Source: CAD feature listing. Evaluate the final solid. Frame: model axes, mm. A direction names the side the tool comes from. Give positions to 0.01 mm unless a question says otherwise; leave off trailing zeros. Write each loop counter-clockwise with the first axis right and the second up, starting at its lowest first coordinate (ties: lowest second). Pieces come first, ordered by that corner, then holes. Notation, with made-up numbers: (68.5, -3) -> (80.5, -3) arc R14 ccw to (80.5, 9) -> close; hole circle Ø3 at (16, 55.5). An arc over 180 degrees is marked (long way). Use one line per item in the form item = value. Start each with the question number.
(1) Cut plane B-B, the plane x = 17.5. Output: boundary loops of the cut face in (y, z), and give its area (3 significant figures).
(2) Draft query along X for faces 4 (the face through (9.56, -6.68, -6.08)), 5 (the face through (26.745, 6.2, 0.1)), 6 (the face through (69.486, -10.648, -13.887)). Return one class per face: pulls with the +X half, pulls with the -X half, needs draft (parallel to the pull), parting line crosses it, or undercut.
(3) Set-up query: faces 1 (the face through (58.381, 0.66, -14.985)), 2 (the face through (50.45, 8.43, 5.38)), 3 (the face through (3.226, 14.756, 9.408)). Return all of +Z, -Z, +X, -X, +Y, -Y with unobstructed straight access to the full face (end or side cutting, diameter ignored); none if empty.
(4) Cut plane A-A, the plane x = 55. Output: boundary loops of the cut face in (y, z).
(5) Material intervals for line 1 along Y through (x, z) = (59, 0); line 2 along X through (y, z) = (-12.5, -7); line 3 along Y through (x, z) = (47.5, 6.5), sorted ascending. Write a range as from..to.
(6) First-contact query: P1, Ø10, axis at x = 64.5, y = 5, coming from the +Z side; P2, Ø6.5, axis at x = 29.5, z = 2, coming from the +Y side; P3, Ø18, axis at x = 17.5, z = 0, coming from the -Y side. Flat tips, straight axial feed; report the tip coordinate or a pass-through.
from build123d import *

# Parameters (mm, degrees)
F2_R     = 15
F3_DEPTH = 19
F4_R     = 10
F5_DEPTH = 25
F6_R     = 1.5


with BuildPart() as f1:
    # F0 (on Front) → F1 (revolve)
    with BuildSketch(Plane.XZ):
        Polygon((0, 17.5), (0, 0), (26.744785, 0), (26.744785, 10), (75, 10), (75, 15), (72, 15), (72, 17.5), (67, 17.5), (67, 15), (50, 15), (5, 17.5), align=None)
    revolve(axis=Axis((13.372393, 0, 0), (-1, 0, 0)))

    # F2 (on Front) → F3 (join)
    with BuildSketch(Plane.XZ):
        with Locations((17.5, 0)):
            Circle(F2_R)
    extrude(amount=F3_DEPTH)

    # F4 (on face) → F5 (cut)
    with BuildSketch(Plane.XZ.offset(19)):
        with Locations((17.5, 0)):
            Circle(F4_R)
    extrude(amount=-F5_DEPTH, mode=Mode.SUBTRACT)

    # F6
    f6_edges = [f1.edges().sort_by_distance(p)[0] for p in [
        (2.5, -19, 0),
        (0, 0, -17.5),
        (67, 0, -17.5),
        (72, 0, -17.5),
        (75, 0, -10),
    ]]
    fillet(f6_edges, radius=F6_R)


solid = f1.part
Geometry says:
q1.outline = (-19, -13.5) arc R1.5 ccw to (-17.5, -15) -> (-7.58, -15) arc R16.81 ccw (long way) to (-7.58, 15) -> (-17.5, 15) arc R1.5 ccw to (-19, 13.5) -> (-19, 10) -> (6, 10) -> (6, -10) -> (-19, -10) -> close
q1.area = 531 mm^2
q2.face_4 = undercut
q2.face_5 = pulls with the +X half
q2.face_6 = needs draft
q3.face_1 = none
q3.face_2 = +X
q3.face_3 = -X
q4.outline = circle Ø30 at (0, 0); hole circle Ø20 at (0, 0)
q5.line_1 = -15..-10, 10..15
q5.line_2 = 0..10.36, 24.64..75
q5.line_3 = -13.67..-7.6, 7.6..13.67
q6.P1 = 17.4
q6.P2 = 16.29
q6.P3 = 6
